from build123d import *

# Parameters (mm, degrees)
F0_DEPTH = 25
F1_R     = 3
F2_DEPTH = 10
F7_DEPTH = 10
F3_DEPTH = 10
F4_R     = 5
F5_R     = 5


with BuildPart() as f0:
    # F6 (on Front) → F0 (new body)
    with BuildSketch(Plane.XZ):
        Polygon((780.004344, -771.129271), (1460.004344, -771.129271), (1460.004344, -731.129271), (1500.004344, -731.129271), (1500.004344, -411.129271), (1460.004344, -411.129271), (1460.004344, -371.129271), (780.004344, -371.129271), (780.004344, -411.129271), (740.004344, -411.129271), (740.004344, -371.129271), (39.646024, -371.129271), (40.004344, -411.127666), (0.004344, -411.127666), (0.004344, -731.13087), (40.004344, -731.13087), (40.361955, -771.129271), (740.004344, -771.129271), (740.004344, -731.129271), (780.004344, -731.129271), align=None)
    extrude(amount=F0_DEPTH)

    # F1 (on face) → F2 (cut)
    with BuildSketch(Plane(origin=(0, 0, 0), x_dir=(-1, 0, 0), z_dir=(0, 1, 0))):
        with Locations((-60.721829, -491.129271)):
            Circle(F1_R)
    extrude(amount=-F2_DEPTH, mode=Mode.SUBTRACT)

    # F1 (on face) → F7 (cut)
    with BuildSketch(Plane(origin=(0, 0, 0), x_dir=(-1, 0, 0), z_dir=(0, 1, 0))):
        with Locations((-59.289877, -651.129271)):
            Circle(F1_R)
    extrude(amount=-F7_DEPTH, mode=Mode.SUBTRACT)

    # F1 (on face) → F3 (cut)
    with BuildSketch(Plane(origin=(0, 0, 0), x_dir=(-1, 0, 0), z_dir=(0, 1, 0))):
        with Locations((-60.721829, -491.129271)):
            Circle(F1_R)
        with Locations((-59.289877, -651.129271)):
            Circle(F1_R)
        with Locations((-1440.004344, -651.129271)):
            Circle(F1_R)
        with Locations((-1440.004344, -491.129271)):
            Circle(F1_R)
    extrude(amount=-F3_DEPTH, mode=Mode.SUBTRACT)

    # F4
    f4_edges = [f0.edges().sort_by_distance(p)[0] for p in [
        (389.825184, -25, -371.129271),
        (390.183149, -25, -771.129271),
    ]]
    fillet(f4_edges, radius=F4_R)

    # F5
    f5_edges = [f0.edges().sort_by_distance(p)[0] for p in [
        (1120.004344, -25, -371.129271),
        (1120.004344, -25, -771.129271),
    ]]
    fillet(f5_edges, radius=F5_R)


solid = f0.part
Model file for the job. Use its own axes, mm. A direction names the side the tool comes from. Round coordinates to 2 decimals unless told otherwise and drop trailing zeros. Loops run counter-clockwise (first coordinate to the right, second up) from the corner with the lowest first, then second, coordinate; pieces in that order, holes last. Notation, with made-up numbers: M -25,36 L 32,36 A16 ccw 32,43 Z; hole C -35.5,12 d2. An arc over 180 degrees is marked long. One line per question, with ' | ' between items.
1) Band-saw the part on A-A (y = -14.5). Give the cut face in (x, z), then the cut area to 3 significant figures.
Solved:
outline: M 0,-731.13 L 40,-731.13 L 40.36,-771.13 L 740,-771.13 L 740,-731.13 L 780,-731.13 L 780,-771.13 L 1460,-771.13 L 1460,-731.13 L 1500,-731.13 L 1500,-411.13 L 1460,-411.13 L 1460,-371.13 L 780,-371.13 L 780,-411.13 L 740,-411.13 L 740,-371.13 L 39.65,-371.13 L 40,-411.13 L 0,-411.13 Z | area: 590,000 mm²
2) Flat gauge pins, fed straight in: pin 1 (5 mm diameter, centred on x = 1440, z = -651.13, fed in from +Y); pin 2 (12.5 mm diameter, centred on y = -17, z = -398, fed in from -X); pin 3 (12.5 mm diameter, centred on y = -6.5, z = -385, fed in from +X). Where does each tip first touch, or does it go through?
Solved:
pin 1: stops at y = -10 | pin 2: stops at x = 39.83 | pin 3: stops at x = 1460
3) 3-axis set-ups, long thin cutter, end or side, ignore diameter. For faces 1 (the flat face through (20, -12, -411.128)), 2 (the flat face through (760, -12, -731.129)), 3 (the flat face through (1460.004, -12, -751)), 4 (the flat face through (760, -12, -411.129)), 5 (the flat face through (1480, -12, -411.129)): which of +Z, -Z, +X, -X, +Y, -Y reach the whole face in a straight line?
Solved:
face 1: +Z, -X, +Y, -Y | face 2: -Z, +Y, -Y | face 3: -Z, +X, +Y, -Y | face 4: +Z, +Y, -Y | face 5: +Z, +X, +Y, -Y
4) Mould opens along X. For faces 6 (the flat face through (740, -25, -568)), 7 (the flat face through (1460.004, -12, -391)), 8 (the flat face through (0.004, -12, -569)), 9 (the flat face through (780.004, -12, -391)) say: +X half, -X half, draft (parallel to the pull), parting line (faces both ways), or undercut.
Solved:
face 6: draft | face 7: +X half | face 8: -X half | face 9: undercut
5) Drill centre lines: line 1 along X through (y, z) = (-16.5, -753); line 2 along X through (y, z) = (-8.5, -652.5); line 3 along Z through (x, y) = (1053, -20.75). Where is each one in solid material? Low to high.
Solved:
line 1: x = 40.2 to 740, 780 to 1460 | line 2: x = 0 to 56.62, 61.96 to 1437.34, 1442.67 to 1500 | line 3: z = -771.07 to -371.19
